Design review of the part built by this model. Coordinates are the model's own, in mm. Coordinates: 2 decimals unless noted, no trailing zeros. Loops run counter-clockwise (first coordinate to the right, second up) from the corner with the lowest first, then second, coordinate; pieces in that order, holes last. Notation, with made-up numbers: (16, -4.5) - (40, -4.5) arc R20 cw to (40, 7.5) - close; hole circle Ø1 at (-20, -7). An arc over 180 degrees is marked (long way). Use one line per item in the form item = value. Start each with the question number.
(1) Add section C-C (z = 2.35). Count the separate pieces of the cut face and the enclosed holes in it, plus the area to 3 significant figures.
(2) Add section A-A (y = 31). State the section outline as (x, z) points, plus the area to 3 significant figures.
(3) For L1, parallel to X at y = -134.5, z = 3.5; L2, parallel to Y at x = -21.5, z = 3.15; L3, parallel to Y at x = 26.5, z = 1.6, list the stretches that pass through material, from the lowest coordinate up.
(4) Add section B-B (x = 8). State the section outline as (y, z) points, plus the area to 3 significant figures.
(5) Clearance check with a flat-ended pin moving along its axis: pin 1 Ø1.6 at (x, y) = (-39, 128) entering from -Z. State where the tip first meets the part, or that it passes through.
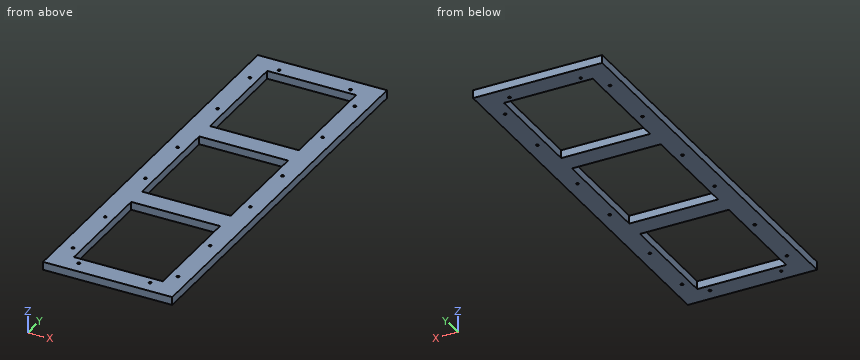
```python
from build123d import *

# Parameters (mm, degrees)
SKETCH1_W           = 96
SKETCH1_H           = 300
SKETCH1_W_2         = 66
SKETCH1_H_2         = 80
BOSS_EXTRUDE1_DEPTH = 6
SKETCH3_R           = 1
CUT_EXTRUDE6_DEPTH  = 10
SKETCH5_R           = 1
CUT_EXTRUDE9_DEPTH  = 10


with BuildPart() as part:
    # Sketch1 → Boss-Extrude1 (new body)
    with BuildSketch(Plane.XY):
        with Locations((0, 6)):
            Rectangle(SKETCH1_W, SKETCH1_H)
        with Locations((0, 101)):
            Rectangle(SKETCH1_W_2, SKETCH1_H_2, mode=Mode.SUBTRACT)
        with Locations((0, -89)):
            Rectangle(SKETCH1_W_2, SKETCH1_H_2, mode=Mode.SUBTRACT)
        with Locations((0, 6)):
            Rectangle(SKETCH1_W_2, SKETCH1_H_2, mode=Mode.SUBTRACT)
    extrude(amount=BOSS_EXTRUDE1_DEPTH)

    # Sketch3 → Cut-Extrude6 (cut)
    with BuildSketch(Plane.XY.offset(6)):
        with Locations((-39, 128)):
            Circle(SKETCH3_R)
        with Locations((-39, 27)):
            Circle(SKETCH3_R)
        with Locations((39, 128)):
            Circle(SKETCH3_R)
        with Locations((39, 83)):
            Circle(SKETCH3_R)
        with Locations((-39, 83)):
            Circle(SKETCH3_R)
        with Locations((39, 27)):
            Circle(SKETCH3_R)
        with Locations((39, -18)):
            Circle(SKETCH3_R)
        with Locations((-39, -18)):
            Circle(SKETCH3_R)
        with Locations((-39, -74)):
            Circle(SKETCH3_R)
        with Locations((39, -74)):
            Circle(SKETCH3_R)
        with Locations((39, -119)):
            Circle(SKETCH3_R)
        with Locations((-39, -119)):
            Circle(SKETCH3_R)
    extrude(amount=-CUT_EXTRUDE6_DEPTH, mode=Mode.SUBTRACT)

    # Sketch5 → Cut-Extrude9 (cut)
    with BuildSketch(Plane.XY.offset(6)):
        with Locations((-26.5, -134.5)):
            Circle(SKETCH5_R)
        with Locations((26.5, -134.5)):
            Circle(SKETCH5_R)
        with Locations((-26.5, 145.5)):
            Circle(SKETCH5_R)
        with Locations((26.5, 145.5)):
            Circle(SKETCH5_R)
    extrude(amount=-CUT_EXTRUDE9_DEPTH, mode=Mode.SUBTRACT)


solid = part.part
```
Computed values:
q1.separate_pieces = 1
q1.enclosed_holes = 19
q1.area = 12,900 mm^2
q2.outline = (-48, 0) - (-33, 0) - (-33, 6) - (-48, 6) - close; (33, 0) - (48, 0) - (48, 6) - (33, 6) - close
q2.area = 180 mm^2
q3.L1 = -48 to -27.5, -25.5 to 25.5, 27.5 to 48
q3.L2 = -144 to -129, -49 to -34, 46 to 61, 141 to 156
q3.L3 = -144 to -135.5, -133.5 to -129, -49 to -34, 46 to 61, 141 to 144.5, 146.5 to 156
q4.outline = (-144, 0) - (-129, 0) - (-129, 6) - (-144, 6) - close; (-49, 0) - (-34, 0) - (-34, 6) - (-49, 6) - close; (46, 0) - (61, 0) - (61, 6) - (46, 6) - close; (141, 0) - (156, 0) - (156, 6) - (141, 6) - close
q4.area = 360 mm^2
q5.pin_1 = through
